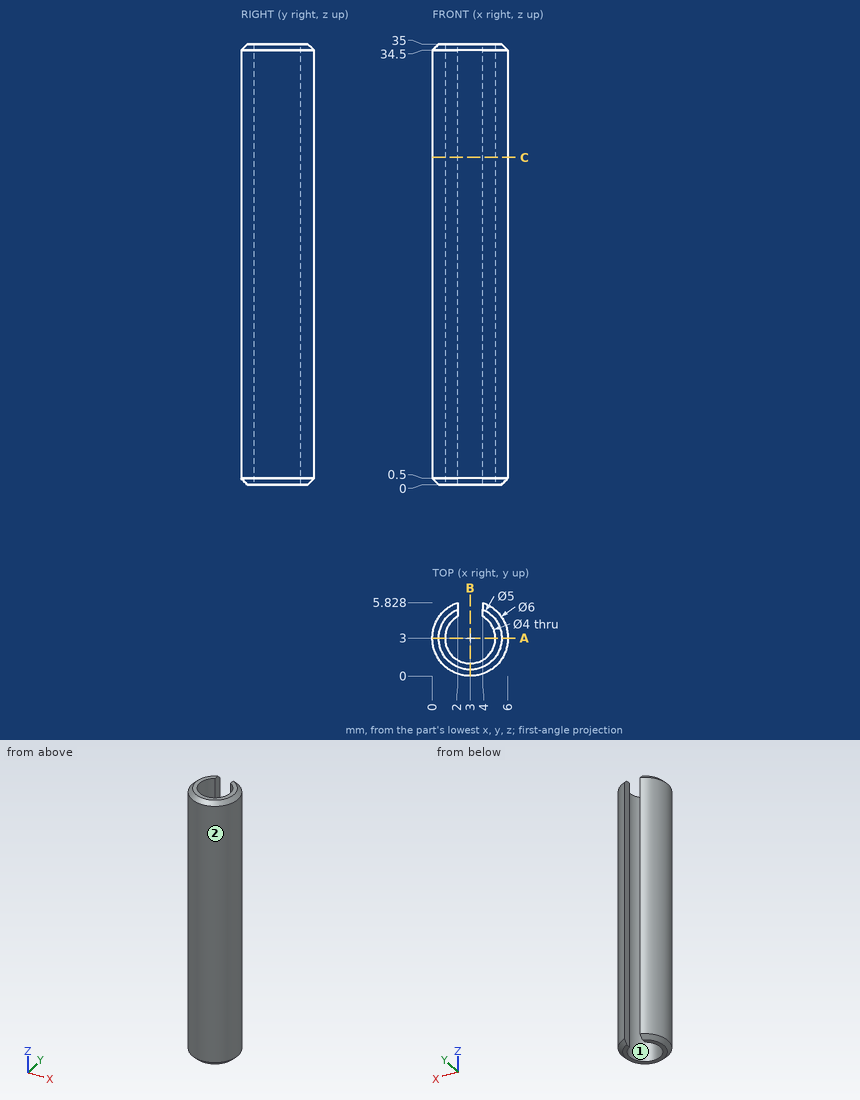
For this review, use the dimensioned drawing (mm, ordinates from the lowest corner) and the shaded views. Round coordinates to 2 decimals unless told otherwise and drop trailing zeros. Write each loop counter-clockwise with the first axis right and the second up, starting at its lowest first coordinate (ties: lowest second). Pieces come first, ordered by that corner, then holes. Notation, with made-up numbers: (55.25, 73) - (112.25, 73) arc R18 cw to (112.25, 102) - close; hole circle Ø4 at (-5, -28.5). An arc over 180 degrees is marked (long way). Answer as a JSON object with one key per item and string values.
1. Draft analysis for pull direction Y (two halves, no side actions). For the marked faces 1 and 2, state which applies: +Y half, -Y half, draft (parallel to the pull), parting line (faces both ways), or undercut.
Response values:
{"face 1": "undercut", "face 2": "parting line"}
2. To check wall thickness, follow line 1 along X through (y, z) = (3.1, 28); line 2 along Y through (x, z) = (3, 17); line 3 along X through (y, z) = (2.55, 9.5) (1 decimal). State the ranges of each line that lie inside material, in increasing order.
Response values:
{"line 1": "x = 0 to 1, 5 to 6", "line 2": "y = 0 to 1", "line 3": "x = 0 to 1.1, 4.9 to 6"}
3. We need section C-C on z = 26. Give the boundary of the cut face in (x, y).
Response values:
{"outline": "(2, 4.73) - (2, 5.83) arc R3 ccw (long way) to (4, 5.83) - (4, 4.73) arc R2 cw (long way) to start"}
4. For pin 1 Ø1 at (x, z) = (4, 21) entering from -Y; pin 2 Ø1.2 at (y, z) = (5.5, 19.5) entering from -X, all flat-tipped, find the tip position at first contact; note any pin that passes through.
Response values:
{"pin 1": "stops at y = 0.04", "pin 2": "stops at x = 0.68"}
5. We need section A-A on y = 3. Give the boundary of the cut face in (x, z).
Response values:
{"outline": "(0, 0.5) - (0.5, 0) - (1, 0) - (1, 35) - (0.5, 35) - (0, 34.5) - close; (5, 0) - (5.5, 0) - (6, 0.5) - (6, 34.5) - (5.5, 35) - (5, 35) - close"}
6. We need section B-B on x = 3. Give the boundary of the cut face in (y, z).
Response values:
{"outline": "(0, 0.5) - (0.5, 0) - (1, 0) - (1, 35) - (0.5, 35) - (0, 34.5) - close"}
